Autodesk Inventor part; units mm, degrees
ref_plane "YZ Plane" through (0, 0, 0) normal (1, 0, 0) x (0, 1, 0)
ref_plane "XZ Plane" through (0, 0, 0) normal (0, 1, 0) x (-1, 0, 0)
ref_plane "XY Plane" through (0, 0, 0) normal (0, 0, 1) x (1, 0, 0)
sketch "スケッチ1" plane through (0, 0, 0) normal (0, 0, 1) x (1, 0, 0)
  line L0 (0, 0) -> (7, 0)
  line L1 (7, 0) -> (7, 20)
  line L2 (7, 20) -> (0, 20)
  line L3 (0, 20) -> (0, 0)
  dimension "d0" = 20
  dimension "d1" = 7
extrude "押し出し1" add sketch "スケッチ1" along normal blind 10
sketch "スケッチ2" plane through (0, 0, 10) normal (0, 0, 1) x (1, 0, 0)
  circle A0 centre (3.5, 15) radius 2.5
  line L0 (0, 0) -> (7, 0)
  line L1 (0, 20) -> (0, 0)
  line L2 (7, 20) -> (0, 20)
  dimension "d4" = 5
  dimension "d6" = 3.5
  dimension "d15" = 5
extrude "押し出し2" cut sketch "スケッチ2" against normal blind 10
sketch "スケッチ3" plane through (0, 0, 0) normal (0, -1, 0) x (1, 0, 0)
  line L0 (33.5, 17) -> (-26.5, 17)
  line L1 (-26.5, 17) -> (-26.5, -7)
  line L2 (-26.5, -7) -> (33.5, -7)
  line L3 (33.5, -7) -> (33.5, 17)
  line L4 (7, 0) -> (0, 0)
  line L5 (3.5, 0) -> (3.5, 10)
  line L6 (0, 10) -> (7, 10)
  line L7 (7, 0) -> (7, 10)
  line L8 (7, 5) -> (0, 5)
  dimension "d9" = 12
  dimension "d10" = 12
  dimension "d11" = 30
  dimension "d12" = 30
extrude "押し出し3" add sketch "スケッチ3" along normal blind 3 contours L3 L2 L1 L0 | L4 L5 L8 L7 | L8 L5 L6 L7
sketch "スケッチ4" plane through (-26.5, 0, 17) normal (0, 0, 1) x (1, 0, 0)
  line L0 (60, 0) -> (0, 0)
  line L1 (0, 0) -> (14, 8.0829)
  line L2 (14, 8.0829) -> (14, 0)
  line L3 (60, 0) -> (46, 8.0829)
  line L4 (46, 8.0829) -> (46, 0)
  point P0 (26.5, 0)
  dimension "d16" = 60
  dimension "d17" = 60
  dimension "d22" = 14
  dimension "d23" = 14
extrude "押し出し4" add sketch "スケッチ4" against normal blind 24
equation "\"d9\" = d10"
equation "\"d11\" = d12"
equation "\"d17\" = d16"
properties part number "sole_practice"
Geometry: final body of the model. Coordinates: model frame, mm. A direction names the side the tool comes from. Coordinates: 2 decimals unless noted, no trailing zeros. Order: outer loops, then holes, each group sorted by start corner. A loop starts at its lowest first (then second) coordinate and runs counter-clockwise, first axis right, second up. Notation, with made-up numbers: (-9, 28.25) -> (39, 28.25) arc R10 ccw to (39, 33.25) -> close; hole circle Ø1 at (24, 63). An arc over 180 degrees is marked (long way). Answer in a Markdown table with one row per item.
Item 1: Section A-A on x = 3.5. Output: boundary loops of the cut face in (y, z).
Return value:
| item | result |
|---|---|
| outline | (-3, -7) -> (0, -7) -> (0, 0) -> (12.5, 0) -> (12.5, 10) -> (0, 10) -> (0, 17) -> (-3, 17) -> close; (17.5, 0) -> (20, 0) -> (20, 10) -> (17.5, 10) -> close |
Item 2: Section D-D on y = 2.75. Output: boundary loops of the cut face in (x, z), plus the area to 3 significant figures.
Return value:
| item | result |
|---|---|
| outline | (-21.74, -7) -> (-12.5, -7) -> (-12.5, 17) -> (-21.74, 17) -> close; (0, 0) -> (7, 0) -> (7, 10) -> (0, 10) -> close; (19.5, -7) -> (28.74, -7) -> (28.74, 17) -> (19.5, 17) -> close |
| area | 513 mm² |
Item 3: Section B-B on y = 15. Output: boundary loops of the cut face in (x, z), plus the area to 3 significant figures.
Return value:
| item | result |
|---|---|
| outline | (0, 0) -> (1, 0) -> (1, 10) -> (0, 10) -> close; (6, 0) -> (7, 0) -> (7, 10) -> (6, 10) -> close |
| area | 20.0 mm² |
Item 4: Contact query for flat-ended pins moving along their axis: P1, Ø6.5, axis at y = 4.5, z = 3.5, coming from the -X side; P2, Ø9, axis at y = 5.5, z = -1, coming from the +X side; P3, Ø12, axis at x = -0.5, y = 13.5, coming from the -Z side. Output: stop coordinate, or through.
Return value:
| item | result |
|---|---|
| P1 | stops at x = -24.33 |
| P2 | stops at x = 31.77 |
| P3 | stops at z = 0 |
Item 5: Access query for faces 4 (the flat face through (3, 10, 10)), 5 (the flat face through (3, 10, 0)), 6 (the flat face through (4, -1, 17)), 7 (the flat face through (19.5, 4, 5)). Directions: +Z, -Z, +X, -X, +Y, -Y. A direction counts if a zero-diameter tool reaches every point of the face in a straight line with its end or side. Return the directions, or none.
Return value:
| item | result |
|---|---|
| face 4 | +Z, +Y |
| face 5 | -Z, +Y |
| face 6 | +Z, +X, -X, +Y, -Y |
| face 7 | +Z, -Z, +Y |
Item 6: Draft query along X for faces 1 (the flat face through (3, -1, -7)), 2 (the flat face through (-26.5, -1, 5)), 3 (the flat face through (0, 10, 5)). Return one class per face: released by +X, released by -X, zero draft, split by the parting line, or undercut.
Return value:
| item | result |
|---|---|
| face 1 | zero draft |
| face 2 | released by -X |
| face 3 | undercut |
Item 7: Section C-C on z = 3.25. Output: boundary loops of the cut face in (x, y), plus the area to 3 significant figures.
Return value:
| item | result |
|---|---|
| outline | (-26.5, -3) -> (33.5, -3) -> (33.5, 0) -> (19.5, 8.08) -> (19.5, 0) -> (7, 0) -> (7, 20) -> (0, 20) -> (0, 0) -> (-12.5, 0) -> (-12.5, 8.08) -> (-26.5, 0) -> close; hole circle Ø5 at (3.5, 15) |
| area | 414 mm² |
Item 8: Ray query, L1, parallel to X at y = 7.75, z = 1.25; L2, parallel to Y at x = 3.5, z = 3.75; L3, parallel to X at y = 4, z = 0.5. Return the intervals inside material, ascending.
Return value:
| item | result |
|---|---|
| L1 | x = -13.08 to -12.5, 0 to 7, 19.5 to 20.08 |
| L2 | y = -3 to 12.5, 17.5 to 20 |
| L3 | x = -19.57 to -12.5, 0 to 7, 19.5 to 26.57 |
